from build123d import *

# Parameters (mm, degrees)
SKETCH1_R           = 8.5
BOSS_EXTRUDE1_DEPTH = 6
SKETCH2_R           = 8.5
BOSS_EXTRUDE2_DEPTH = 6
SKETCH3_R           = 5
SKETCH3_R_2         = 2.75
BOSS_EXTRUDE3_DEPTH = 5
SKETCH4_W           = 28
SKETCH4_H           = 5
BOSS_EXTRUDE5_DEPTH = 47
FILLET1_R           = 2


with BuildPart() as part:
    # Sketch1 → Boss-Extrude1 (new body)
    with BuildSketch(Plane.XY):
        with BuildLine():
            Line((14, -16), (14, 0))
            ThreePointArc((14, 0), (0, 14), (-14, 0))
            Line((-14, 0), (-14, -16))
            Line((-14, -16), (14, -16))
        make_face()
        Circle(SKETCH1_R, mode=Mode.SUBTRACT)
    extrude(amount=BOSS_EXTRUDE1_DEPTH)



with BuildPart() as body_2:
    # Sketch2 → Boss-Extrude2 (new body)
    with BuildSketch(Plane(origin=(0, 0, -15), x_dir=(-1, 0, 0), z_dir=(0, 0, -1))):
        with BuildLine():
            Line((-14, -16), (-14, 0))
            ThreePointArc((-14, 0), (0, 14), (14, 0))
            Line((14, 0), (14, -16))
            Line((14, -16), (-14, -16))
        make_face()
        with Locations(Location((0, 0, 0), (0, 0, 180))):
            Circle(SKETCH2_R, mode=Mode.SUBTRACT)
    extrude(amount=BOSS_EXTRUDE2_DEPTH)


with BuildPart() as body_3:
    # Sketch3 → Boss-Extrude3 (new body)
    with BuildSketch(Plane(origin=(0, 0, -26), x_dir=(-1, 0, 0), z_dir=(0, 0, -1))):
        with BuildLine():
            Line((-14, -16), (14, -16))
            Line((14, -16), (14, 0))
            ThreePointArc((14, 0), (0, 14), (-14, 0))
            Line((-14, 0), (-14, -16))
        make_face()
        Circle(SKETCH3_R, mode=Mode.SUBTRACT)
        with Locations((-10, 0)):
            Circle(SKETCH3_R_2, mode=Mode.SUBTRACT)
        with Locations((10, 0)):
            Circle(SKETCH3_R_2, mode=Mode.SUBTRACT)
    extrude(amount=BOSS_EXTRUDE3_DEPTH)


with BuildPart() as part_1:
    add(part.part)

    add(body_2.part)  # Boss-Extrude5 merges body 2

    add(body_3.part)  # Boss-Extrude5 merges body 3
    # Sketch4 → Boss-Extrude5 (add)
    with BuildSketch(Plane.XY.offset(6)):
        with Locations((0, -18.5)):
            Rectangle(SKETCH4_W, SKETCH4_H)
    extrude(amount=-BOSS_EXTRUDE5_DEPTH)

    # Fillet1
    fillet1_edges = [part_1.edges().sort_by_distance(p)[0] for p in [
        (0, -21, 6),
        (14, -18.5, -41),
        (-14, -18.5, -41),
        (0, -16, -21),
        (0, -16, -15),
        (0, -16, -26),
        (0, -16, 0),
    ]]
    fillet(fillet1_edges, radius=FILLET1_R)


solid = part_1.part
Input: part model. Units: mm. Frame: model coordinates. A direction names the side the tool comes from. Round coordinates to 2 decimals unless told otherwise and drop trailing zeros. Order: outer loops, then holes, each group sorted by start corner. A loop starts at its lowest first (then second) coordinate and runs counter-clockwise, first axis right, second up. Notation, with made-up numbers: (65.25, -25) - (118.25, -25) arc R7 cw to (118.25, -18) - close; hole circle Ø7 at (0.25, -17). An arc over 180 degrees is marked (long way). Answer as a JSON object with one key per item and string values. Group by question number.
(1) Reachability of faces 4 (the face through (-1.107, -8.428, -17.958)), 5 (the face through (-12.54, -1.05, -28.46)), 6 (the face through (0.2, -15.4, -21.57)), 7 (the face through (3.3, -4.1, -31)), 8 (the face through (-14, -13, -16)) from +Z, -Z, +X, -X, +Y, -Y: full face, straight path, thin tool, end or side. Return the list, or none.
(2) Draft query along X for faces 1 (the face through (0.2, -15.43, -14.4)), 2 (the face through (-13.43, -18.46, -40.4)), 3 (the face through (7.46, -1.05, -28.46)). Return one class per face: released by +X, released by -X, zero draft, split by the parting line, or undercut.
(3) Cut plane D-D (x = -11.25). Return loops of the section in (y, z).
(4) Pin query (flat end, axial travel): P1, Ø1.5, axis at x = 11, z = -3.5, coming from the +Y side; P2, Ø4, axis at x = -10, z = -15.5, coming from the +Y side; P3, Ø2, axis at x = -4, y = -10.5, coming from the -Z side; P4, Ø2, axis at y = -15, z = -22.5, coming from the -X side. Return the tip coordinate at first contact, or that it passes through.
(5) Material intervals for probe 1 along Z at (x, y) = (-11, -12.5); probe 2 along Y at (x, z) = (0, -27.95); probe 3 along Y at (x, z) = (0, -18.8), sorted ascending. Write a range as from..to.
(6) Cut plane C-C (y = -13). Return loops of the section in (x, z), then the cut area to 3 significant figures.
(7) Cut plane B-B (x = -4.25). Count the separate pieces of the cut face and the enclosed holes in it, then the cut area to 3 significant figures.
(8) Cut plane A-A (y = -7.5). Return loops of the section in (x, z), then the cut area to 3 significant figures.
Here are the results:
{
 "1": {"face 4": "+Z", "face 5": "-Z", "face 6": "+X, -X, +Y", "face 7": "-Z, +X, -X, +Y", "face 8": "+Z, -Z, -X, +Y, -Y"},
 "2": {"face 1": "zero draft", "face 2": "released by -X", "face 3": "undercut"},
 "3": {"outline": "(-21, -41) - (-16, -41) - (-16, -31) - (-2.45, -31) - (-2.45, -26) - (-14, -26) arc R2 cw to (-16, -24) - (-16, -23) arc R2 cw to (-14, -21) - (8.33, -21) - (8.33, -15) - (-14, -15) arc R2 cw to (-16, -13) - (-16, -2) arc R2 cw to (-14, 0) - (8.33, 0) - (8.33, 6) - (-19, 6) arc R2 ccw to (-21, 4) - close; (2.45, -31) - (8.33, -31) - (8.33, -26) - (2.45, -26) - close"},
 "4": {"P1": "stops at y = -16", "P2": "stops at y = 11.49", "P3": "stops at z = -31", "P4": "stops at x = -14"},
 "5": {"probe 1": "z = -31..-26, -21..-15, 0..6", "probe 2": "y = -21..-5, 5..14", "probe 3": "y = -21..-8.5, 8.5..14"},
 "6": {"outline": "(-14, -31) - (14, -31) - (14, -26) - (-14, -26) - close; (-14, -21) - (14, -21) - (14, -15) - (-14, -15) - close; (-14, 0) - (14, 0) - (14, 6) - (-14, 6) - close", "area": "476 mm^2"},
 "7": {"separate pieces": "4", "enclosed holes": "0", "area": "533 mm^2"},
 "8": {"outline": "(-14, -31) - (14, -31) - (14, -26) - (-14, -26) - close; (-14, -21) - (-4, -21) - (-4, -15) - (-14, -15) - close; (-14, 0) - (-4, 0) - (-4, 6) - (-14, 6) - close; (4, -21) - (14, -21) - (14, -15) - (4, -15) - close; (4, 0) - (14, 0) - (14, 6) - (4, 6) - close", "area": "380 mm^2"}
}
